Geometry check sheet. Reference: the model listing, model coordinates, mm. Face numbers are marked on the shaded views. A direction names the side the tool comes from. Give positions to 0.01 mm unless a question says otherwise; leave off trailing zeros. Loops run counter-clockwise (first coordinate to the right, second up) from the corner with the lowest first, then second, coordinate; pieces in that order, holes last. Notation, with made-up numbers: (-16, 13.25) - (13, 13.25) arc R27 ccw to (13, 43.25) - close; hole circle Ø10 at (12, 2). An arc over 180 degrees is marked (long way). Write item = value, one per line. Start each with the question number.
from build123d import *

# Parameters (mm, degrees)
F0_W     = 15.75
F0_H     = 15.75
F0_W_2   = 0.6
F0_H_2   = 0.37
F0_W_3   = 0.37
F0_H_3   = 0.6
F1_DEPTH = 9.55
F0_R     = 3.3
F0_R_2   = 2.5
F2_DEPTH = 1.55
F4_DEPTH = 1.9


with BuildPart() as f1:
    # F0 (on Top) → F1 (new body)
    with BuildSketch(Plane.XY):
        with Locations((7.875, 7.875)):
            Rectangle(F0_W, F0_H)
        Polygon((1.13, 12.225), (1.13, 14.62), (3.525, 14.62), (4.125, 14.62), (11.625, 14.62), (12.225, 14.62), (14.62, 14.62), (14.62, 12.225), (14.62, 11.625), (14.62, 4.125), (14.62, 3.525), (14.62, 1.13), (12.225, 1.13), (11.625, 1.13), (4.125, 1.13), (3.525, 1.13), (1.13, 1.13), (1.13, 3.525), (1.13, 4.125), (1.13, 11.625), align=None, mode=Mode.SUBTRACT)
        with Locations((3.825, 14.435)):
            Rectangle(F0_W_2, F0_H_2)
        with Locations((1.315, 11.925)):
            Rectangle(F0_W_3, F0_H_3)
        with Locations((1.315, 3.825)):
            Rectangle(F0_W_3, F0_H_3)
        with Locations((3.825, 1.315)):
            Rectangle(F0_W_2, F0_H_2)
        with Locations((11.925, 1.315)):
            Rectangle(F0_W_2, F0_H_2)
        with Locations((14.435, 3.825)):
            Rectangle(F0_W_3, F0_H_3)
        with Locations((14.435, 11.925)):
            Rectangle(F0_W_3, F0_H_3)
        with Locations((11.925, 14.435)):
            Rectangle(F0_W_2, F0_H_2)
    extrude(amount=F1_DEPTH)



with BuildPart() as f1b:
    # F0 (on Top) → F1, piece 2 (new body)
    with BuildSketch(Plane.XY):
        with Locations((7.875, 7.875)):
            Circle(F0_R)
        with Locations((7.875, 7.875)):
            Circle(F0_R_2, mode=Mode.SUBTRACT)
    extrude(amount=F1_DEPTH)


with BuildPart() as f1_1:
    add(f1.part)

    add(f1b.part)  # F2 merges F1b
    # F0 (on Top) → F2 (join)
    with BuildSketch(Plane.XY):
        Polygon((3.525, 14.62), (1.13, 14.62), (1.13, 12.225), (1.5, 12.225), (1.5, 11.625), (1.13, 11.625), (1.13, 4.125), (1.5, 4.125), (1.5, 3.525), (1.13, 3.525), (1.13, 1.13), (3.525, 1.13), (3.525, 1.5), (4.125, 1.5), (4.125, 1.13), (11.625, 1.13), (11.625, 1.5), (12.225, 1.5), (12.225, 1.13), (14.62, 1.13), (14.62, 3.525), (14.25, 3.525), (14.25, 4.125), (14.62, 4.125), (14.62, 11.625), (14.25, 11.625), (14.25, 12.225), (14.62, 12.225), (14.62, 14.62), (12.225, 14.62), (12.225, 14.25), (11.625, 14.25), (11.625, 14.62), (4.125, 14.62), (4.125, 14.25), (3.525, 14.25), align=None)
        with Locations((7.875, 7.875)):
            Circle(F0_R, mode=Mode.SUBTRACT)
        with Locations((7.875, 7.875)):
            Circle(F0_R_2)
    extrude(amount=F2_DEPTH)

    # F3 (on face) → F4 (join)
    with BuildSketch(Plane.XY):
        with BuildLine():
            ThreePointArc((5.1239527498, 6.0524361391), (1.8449210985, 2.7120455778), (6.3625, 3.9375))
            ThreePointArc((6.3625, 3.9375), (6.2837038634, 4.5506495995), (6.0524361391, 5.1239527498))
            ThreePointArc((6.0524361391, 5.1239527498), (5.5415476221, 5.5415476221), (5.1239527498, 6.0524361391))
        make_face()
        with BuildLine():
            ThreePointArc((10.6260472502, 6.0524361391), (10.2084523779, 5.5415476221), (9.6975638609, 5.1239527498))
            ThreePointArc((9.6975638609, 5.1239527498), (11.1993504005, 1.5912961366), (14.2375, 3.9375))
            ThreePointArc((14.2375, 3.9375), (13.0379544222, 6.0300789015), (10.6260472502, 6.0524361391))
        make_face()
        with BuildLine():
            ThreePointArc((6.3625, 11.8125), (1.8449210985, 13.0379544222), (5.1239527498, 9.6975638609))
            ThreePointArc((5.1239527498, 9.6975638609), (5.5415476221, 10.2084523779), (6.0524361391, 10.6260472502))
            ThreePointArc((6.0524361391, 10.6260472502), (6.2837038634, 11.1993504005), (6.3625, 11.8125))
        make_face()
        with BuildLine():
            ThreePointArc((14.2375, 11.8125), (11.1993504005, 14.1587038634), (9.6975638609, 10.6260472502))
            ThreePointArc((9.6975638609, 10.6260472502), (10.2084523779, 10.2084523779), (10.6260472502, 9.6975638609))
            ThreePointArc((10.6260472502, 9.6975638609), (13.0379544222, 9.7199210985), (14.2375, 11.8125))
        make_face()
    extrude(amount=-F4_DEPTH)


solid = f1_1.part
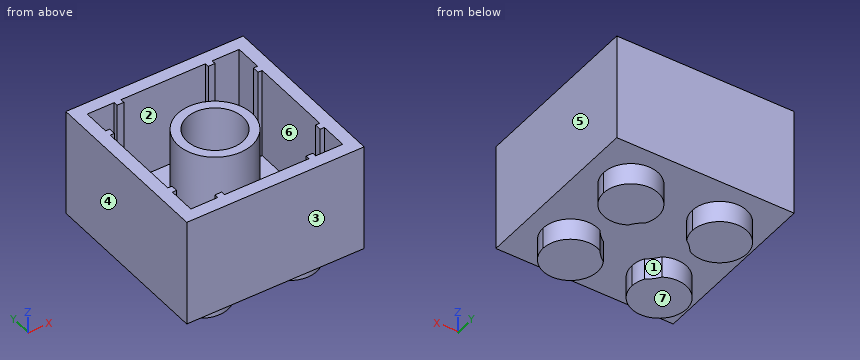
1) Release check for a two-part mould opening along X. For the marked faces 4, 5, 6 and 7 record: pulls with the +X half, pulls with the -X half, needs draft (parallel to the pull), parting line crosses it, or undercut.
2) Cross-section at A-A on z = -1. Give the number of separate pieces and of enclosed holes in the cut face, and give its area (3 significant figures).
3) Cross-section at C-C on y = 7. Enter the section's corners in (x, z).
4) Gauge pin test, flat end, axial feed: P1, Ø4, axis at y = 7, z = 1, coming from the -X side. Record the tip position at first contact, or that the pin passes through.
5) Material ranges on line 1 along X through (y, z) = (14.5, 3) (3 decimals); line 2 along Y through (x, z) = (5.75, 9.25); line 3 along Y through (x, z) = (11.25, 4.25), recorded low to high.
6) Tool access check on the marked faces 1, 2 and 3. Record the directions out of +Z, -Z, +X, -X, +Y, -Y that give a thin tool (end or side, any length) a straight path to the whole face; none if there is none.
7) Cross-section at B-B on x = 7.75. Enter the section's corners in (y, z), and give its area (3 significant figures).
Checked values:
q1.face_4 = pulls with the -X half
q1.face_5 = pulls with the +X half
q1.face_6 = undercut
q1.face_7 = needs draft
q2.separate_pieces = 4
q2.enclosed_holes = 0
q2.area = 73.3 mm²
q3.outline = (0, 0) - (15.75, 0) - (15.75, 9.55) - (14.62, 9.55) - (14.62, 1.55) - (11.06, 1.55) - (11.06, 9.55) - (10.22, 9.55) - (10.22, 1.55) - (5.53, 1.55) - (5.53, 9.55) - (4.69, 9.55) - (4.69, 1.55) - (1.13, 1.55) - (1.13, 9.55) - (0, 9.55) - close
q4.P1 = 0
q5.line_1 = 0 to 1.13, 3.525 to 4.125, 11.625 to 12.225, 14.62 to 15.75
q5.line_2 = 0 to 1.13, 5.35 to 6.56, 9.19 to 10.4, 14.62 to 15.75
q5.line_3 = 0 to 1.13, 14.62 to 15.75
q6.face_1 = -Z
q6.face_2 = +Z
q6.face_3 = +Z, -Z, +X, -X, -Y
q7.outline = (0, 0) - (15.75, 0) - (15.75, 9.55) - (14.62, 9.55) - (14.62, 1.55) - (11.17, 1.55) - (11.17, 9.55) - (10.37, 9.55) - (10.37, 1.55) - (5.38, 1.55) - (5.38, 9.55) - (4.58, 9.55) - (4.58, 1.55) - (1.13, 1.55) - (1.13, 9.55) - (0, 9.55) - close
q7.area = 55.3 mm²
